from build123d import *

# Parameters (mm, degrees)
SKETCH1_W                                        = 74
SKETCH1_H                                        = 52
EXTRUDE1_DEPTH                                   = 20
CSK_FOR_M10_FLAT_HEAD_MACHINE_SCREW1_D           = 11
CSK_FOR_M10_FLAT_HEAD_MACHINE_SCREW1_CSINK_D     = 20
CSK_FOR_M10_FLAT_HEAD_MACHINE_SCREW1_CSINK_ANGLE = 90
F_8_0_8_DIAMETER_HOLE1_D                         = 8
CBORE_FOR_M8_SHCS1_D                             = 9
CBORE_FOR_M8_SHCS1_CBORE_D                       = 15
CBORE_FOR_M8_SHCS1_CBORE_DEPTH                   = 8
SKETCH8_R                                        = 8
CUT_EXTRUDE1_DEPTH                               = 6


with BuildPart() as part:
    # Sketch1 → Extrude1 (new body)
    with BuildSketch(Plane(origin=(0, 0, 0), x_dir=(1, 0, 0), z_dir=(0, 1, 0))):
        with Locations((5, 0)):
            Rectangle(SKETCH1_W, SKETCH1_H)
    extrude(amount=EXTRUDE1_DEPTH)

    # CSK for M10 Flat Head Machine Screw1 (through all)
    with Locations(Plane(origin=(0, 20, 0), x_dir=(-1, 0, 0), z_dir=(0, 1, 0))):
        with Locations((-27, 0)):
            CounterSinkHole(CSK_FOR_M10_FLAT_HEAD_MACHINE_SCREW1_D / 2, CSK_FOR_M10_FLAT_HEAD_MACHINE_SCREW1_CSINK_D / 2, counter_sink_angle=CSK_FOR_M10_FLAT_HEAD_MACHINE_SCREW1_CSINK_ANGLE)

    # Ø8.0 (8) Diameter Hole1 (through all)
    with Locations(Plane(origin=(0, 20, 0), x_dir=(-1, 0, 0), z_dir=(0, 1, 0))):
        with Locations((0, -13)):
            Hole(F_8_0_8_DIAMETER_HOLE1_D / 2)

    # CBORE for M8 SHCS1 (through all)
    with Locations(Plane.XZ):
        with Locations((-20, 14)):
            CounterBoreHole(CBORE_FOR_M8_SHCS1_D / 2, CBORE_FOR_M8_SHCS1_CBORE_D / 2, CBORE_FOR_M8_SHCS1_CBORE_DEPTH)

    # Sketch8 → Cut-Extrude1 (cut)
    with BuildSketch(Plane(origin=(0, 13, 0), x_dir=(-1, 0, 0), z_dir=(0, 1, 0))):
        with Locations(Location((0, -13, 0), (0, 0, 90))):
            Circle(SKETCH8_R)
    extrude(amount=-CUT_EXTRUDE1_DEPTH, mode=Mode.SUBTRACT)


solid = part.part
Source: CAD feature listing. Evaluate the final solid. Frame: model axes, mm. A direction names the side the tool comes from. Give positions to 0.01 mm unless a question says otherwise; leave off trailing zeros. Write each loop counter-clockwise with the first axis right and the second up, starting at its lowest first coordinate (ties: lowest second). Pieces come first, ordered by that corner, then holes. Notation, with made-up numbers: (-19.5, 23.5) - (5.5, 23.5) arc R24 cw to (5.5, 51.5) - close; hole circle Ø4 at (64, 86.25). An arc over 180 degrees is marked (long way). Write item = value, one per line. Start each with the question number.
Q1. Pin query (flat end, axial travel): pin 1 Ø5 at (x, z) = (-1, -13.5) entering from -Y; pin 2 Ø11.5 at (x, z) = (-20, 14) entering from -Y. Return the tip coordinate at first contact, or that it passes through.
Q2. Cut plane C-C, the plane x = 27. Return loops of the section in (y, z).
Q3. Cut plane B-B, the plane y = 17.5. Return loops of the section in (x, z), then the cut area to 3 significant figures.
Q4. Cut plane A-A, the plane z = 0. Return loops of the section in (x, y), then the cut area to 3 significant figures.
Q5. Cut plane D-D, the plane z = -13. Return loops of the section in (x, y).
Q6. Material intervals for probe 1 along Z at (x, y) = (-20, 2.75); probe 2 along Z at (x, y) = (0, 4.5); probe 3 along X at (y, z) = (13.25, 5), sorted ascending.
Q7. Draft query along Y for faces 4 (the flat face through (4, 10, 26)), 5 (the flat face through (4, 0, 0)), 6 (the flat face through (-2, 13, -17)). Return one class per face: +Y half, -Y half, draft (parallel to the pull), parting line (faces both ways), or undercut.
Q8. Reachability of faces 1 (the cylindrical face through (-7.81, 10.04, -14.73)), 2 (the conical face through (22.5, 15.7, -3.5)), 3 (the cylindrical face through (-25.952, 3.944, 9.436)) from +Z, -Z, +X, -X, +Y, -Y: full face, straight path, thin tool, end or side. Return the list, or none.
Computed values:
q1.pin_1 = through
q1.pin_2 = 8
q2.outline = (0, -26) - (20, -26) - (20, -10) - (15.5, -5.5) - (0, -5.5) - close; (0, 5.5) - (15.5, 5.5) - (20, 10) - (20, 26) - (0, 26) - close
q3.outline = (-32, -26) - (42, -26) - (42, 26) - (-32, 26) - close; hole circle Ø9 at (-20, 14); hole circle Ø8 at (0, -13); hole circle Ø15 at (27, 0)
q3.area = 3,560 mm²
q4.outline = (-32, 0) - (21.5, 0) - (21.5, 15.5) - (17, 20) - (-32, 20) - close; (32.5, 0) - (42, 0) - (42, 20) - (37, 20) - (32.5, 15.5) - close
q4.area = 1,240 mm²
q5.outline = (-32, 0) - (-4, 0) - (-4, 7) - (-8, 7) - (-8, 13) - (-4, 13) - (-4, 20) - (-32, 20) - close; (4, 0) - (42, 0) - (42, 20) - (4, 20) - (4, 13) - (8, 13) - (8, 7) - (4, 7) - close
q6.probe_1 = -26 to 6.5, 21.5 to 26
q6.probe_2 = -26 to -17, -9 to 26
q6.probe_3 = -32 to 24.71, 29.29 to 42
q7.face_4 = draft
q7.face_5 = -Y half
q7.face_6 = undercut
q8.face_1 = none
q8.face_2 = +Y
q8.face_3 = -Y
